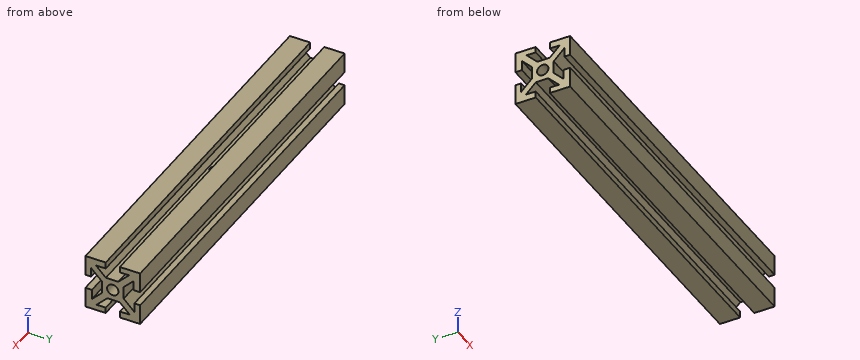
from build123d import *

# Parameters (mm, degrees)
SKETCH1_W           = 10
SKETCH1_H           = 10
SKETCH1_R           = 2.605
BOSS_EXTRUDE1_DEPTH = 172.72
CIRPATTERN1_COUNT   = 4
SKETCH2_R           = 2.38
CUT_EXTRUDE6_DEPTH  = 8


with BuildPart() as part:
    # Sketch1 → Boss-Extrude1 (new body)
    with BuildSketch(Plane(origin=(0, 0, 0), x_dir=(0, 0, -1), z_dir=(1, 0, 0))):
        Rectangle(SKETCH1_W, SKETCH1_H)
        Circle(SKETCH1_R, mode=Mode.SUBTRACT)
        Polygon((7.474873734, 9.921463197), (2.553410537, 5), (5, 5), (5, 3.203948776), (9.596194078, 7.800142853), align=None)
        Polygon((9.596194078, 3.24), (12.596194078, 3.24), (12.596194078, 12.596194078), (3.24, 12.596194078), (3.24, 9.921463197), (7.474873734, 9.921463197), (9.596194078, 7.800142853), align=None)
    boss_extrude1 = extrude(amount=BOSS_EXTRUDE1_DEPTH)

    # CirPattern1: Boss-Extrude1 ×4 about axis
    cirpattern1_axis = Axis((0, 0, 0), (1, 0, 0))
    for i in range(1, CIRPATTERN1_COUNT):
        add(boss_extrude1.rotate(cirpattern1_axis, i * 360 / CIRPATTERN1_COUNT))

    # Sketch2 → Cut-Extrude6 (cut)
    with BuildSketch(Plane.XY.offset(12.596194078)):
        with Locations((86.36, 0)):
            Circle(SKETCH2_R)
    extrude(amount=-CUT_EXTRUDE6_DEPTH, mode=Mode.SUBTRACT)


solid = part.part
Read the model definition and answer for the solid it produces. Units are mm, in the model's axes. Round coordinates to 2 decimals unless told otherwise and drop trailing zeros. Loops run counter-clockwise (first coordinate to the right, second up) from the corner with the lowest first, then second, coordinate; pieces in that order, holes last.
Q1. Each of these flat-tipped pins is pushed along its axis until it touches: pin 1 (4.5 mm diameter, centred on y = 0, z = 0, fed in from -X); pin 2 (4 mm diameter, centred on x = 85.5, y = 1, fed in from +Z); pin 3 (3 mm diameter, centred on x = 91.5, z = 0, fed in from -Y). Where does it stop, or does it pass through?
Q2. Section A-A on y = 0 is taken. Write down the section's boundary in (x, z) (3 decimals), and give its area (3 significant figures).
Q3. Section B-B on z = 0 is taken. Write down the section's boundary in (x, y) (3 decimals), and give its area (3 significant figures).
Q4. Consider probe 1 along Y at (x, z) = (124, -10.5); probe 2 along Y at (x, z) = (58, 0) (3 decimals); probe 3 along Y at (x, z) = (33, 7.25). Determine where each line is inside the solid, lowest interval first.
Output:
1. pin 1: passes through
1. pin 2: stops at z = 5.45
1. pin 3: stops at y = -5
2. outline: (0, -5) - (172.72, -5) - (172.72, -2.605) - (0, -2.605) - close; (0, 2.605) - (172.72, 2.605) - (172.72, 5) - (88.74, 5) - (88.74, 4.596) - (83.98, 4.596) - (83.98, 5) - (0, 5) - close
2. area: 825 mm2
3. outline: (0, -5) - (172.72, -5) - (172.72, -2.605) - (0, -2.605) - close; (0, 2.605) - (172.72, 2.605) - (172.72, 5) - (0, 5) - close
3. area: 827 mm2
4. probe 1: y = -12.6 to -3.24, 3.24 to 12.6
4. probe 2: y = -5 to -2.605, 2.605 to 5
4. probe 3: y = -12.6 to -9.92, -9.7 to -5.45, 4.8 to 9.05, 9.6 to 12.6
